The listing builds one solid part. Answer for the finished solid, in the listing's coordinates (mm). Face numbers are marked on the shaded views. A direction names the side the tool comes from. Round coordinates to 2 decimals unless told otherwise and drop trailing zeros. Order: outer loops, then holes, each group sorted by start corner. A loop starts at its lowest first (then second) coordinate and runs counter-clockwise, first axis right, second up. Notation, with made-up numbers: M 87.5,85 L 130.5,85 A21 cw 130.5,97 Z; hole C 68,47.5 d10. An arc over 180 degrees is marked long. Write item = value, one per line. Start each with the question number.
(1) Which of the six approach directions +Z, -Z, +X, -X, +Y, -Y give full straight-line access (tool end or side, diameter ignored) to the marked faces 1 and 2?
(2) A cutting plane is placed at B-B, the plane z = -12. Determine the outline of the cut face in (x, y).
(3) For a pull along Z with two mould halves and no side action, classify the marked faces 3, 4 and 5 as released by +Z, released by -Z, zero draft, split by the parting line, or undercut.
(4) This flat-tipped pin is pushed along its axis until it touches: pin 1 (3.5 mm diameter, centred on x = 32, z = -12, fed in from -Y). Where does it stop, or does it pass through?
(5) Straight lines are drawn through the part: probe 1 along X at (y, z) = (12.8, -12); probe 2 along X at (y, z) = (3, -12); probe 3 along Z at (x, y) = (32, 4). For each, find the intervals that lie inside material, in ascending order. Write a range as from..to.
(6) A cutting plane is placed at A-A, the plane x = 4. Determine the outline of the cut face in (y, z), and give its area (3 significant figures).
(7) A cutting plane is placed at D-D, the plane y = 2.25. Determine the outline of the cut face in (x, z), and give its area (3 significant figures).
(8) A cutting plane is placed at C-C, the plane y = 11.75. Determine the outline of the cut face in (x, z).
from build123d import *

# Parameters (mm, degrees)
SKETCH1_W                  = 36
SKETCH1_H                  = 24
BOSS_EXTRUDE1_DEPTH        = 15
SKETCH2_R                  = 8
CUT_EXTRUDE1_DEPTH         = 5
F_3_2_3_2_DIAMETER_HOLE1_D = 3.2


with BuildPart() as part:
    # Sketch1 → Boss-Extrude1 (new body)
    with BuildSketch(Plane(origin=(0, 0, 0), x_dir=(1, 0, 0), z_dir=(0, 1, 0))):
        with Locations((18, 12)):
            Rectangle(SKETCH1_W, SKETCH1_H)
    extrude(amount=BOSS_EXTRUDE1_DEPTH)

    # Sketch2 → Cut-Extrude1 (cut)
    with BuildSketch(Plane(origin=(0, 15, 0), x_dir=(1, 0, 0), z_dir=(0, 1, 0))):
        with Locations(Location((18, 12, 0), (0, 0, 270))):
            Circle(SKETCH2_R)
    extrude(amount=-CUT_EXTRUDE1_DEPTH, mode=Mode.SUBTRACT)

    # Ø3.2 (3.2) Diameter Hole1 (through all)
    with Locations(Plane(origin=(0, 15, 0), x_dir=(1, 0, 0), z_dir=(0, 1, 0))):
        with Locations((4, 12), (32, 12)):
            Hole(F_3_2_3_2_DIAMETER_HOLE1_D / 2)


solid = part.part
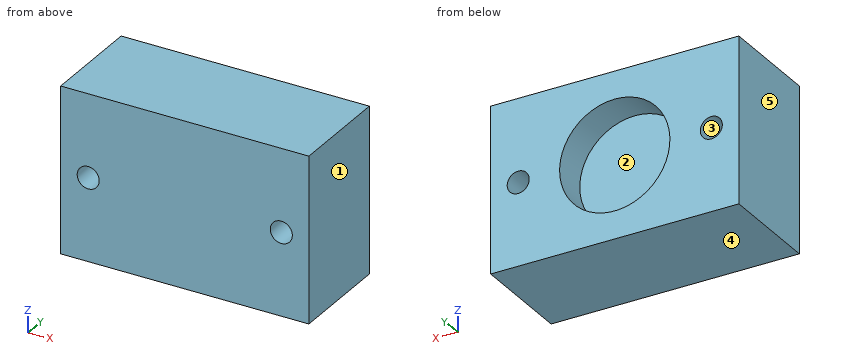
Reported:
q1.face_1 = +Z, -Z, +X, +Y, -Y
q1.face_2 = +Y
q2.outline = M 0,0 L 2.4,0 L 2.4,15 L 0,15 Z; M 5.6,0 L 30.4,0 L 30.4,15 L 26,15 L 26,10 L 10,10 L 10,15 L 5.6,15 Z; M 33.6,0 L 36,0 L 36,15 L 33.6,15 Z
q3.face_3 = undercut
q3.face_4 = released by -Z
q3.face_5 = zero draft
q4.pin_1 = 0
q5.probe_1 = 0..2.4, 5.6..10, 26..30.4, 33.6..36
q5.probe_2 = 0..2.4, 5.6..30.4, 33.6..36
q5.probe_3 = -24..-13.6, -10.4..0
q6.outline = M 0,-24 L 15,-24 L 15,-13.6 L 0,-13.6 Z; M 0,-10.4 L 15,-10.4 L 15,0 L 0,0 Z
q6.area = 312 mm²
q7.outline = M 0,-24 L 36,-24 L 36,0 L 0,0 Z; hole C 4,-12 d3.2; hole C 32,-12 d3.2
q7.area = 848 mm²
q8.outline = M 0,-24 L 36,-24 L 36,0 L 0,0 Z; hole C 4,-12 d3.2; hole C 18,-12 d16; hole C 32,-12 d3.2
